```python
from build123d import *

# Parameters (mm, degrees)
SKETCH10_W          = 150
SKETCH10_H          = 150
BOSS_EXTRUDE3_DEPTH = 10
SKETCH12_W          = 100
SKETCH12_H          = 37.5
CUT_EXTRUDE2_DEPTH  = 10
FILLET7_R           = 10


with BuildPart() as part:
    # Sketch10 → Boss-Extrude3 (new body)
    with BuildSketch(Plane(origin=(0, 0, 0), x_dir=(0, 0, -1), z_dir=(1, 0, 0))):
        with Locations((75, 112.5)):
            Rectangle(SKETCH10_W, SKETCH10_H)
    extrude(amount=BOSS_EXTRUDE3_DEPTH)

    # Sketch12 → Cut-Extrude2 (cut)
    with BuildSketch(Plane.ZY):
        with Locations((-75, 56.25)):
            Rectangle(SKETCH12_W, SKETCH12_H)
    extrude(amount=-CUT_EXTRUDE2_DEPTH, mode=Mode.SUBTRACT)

    # Fillet7
    fillet7_edges = [part.edges().sort_by_distance(p)[0] for p in [
        (5, 37.5, -125),
        (5, 37.5, -25),
        (5, 187.5, 0),
        (5, 187.5, -150),
        (5, 37.5, -150),
        (5, 37.5, 0),
    ]]
    fillet(fillet7_edges, radius=FILLET7_R)


solid = part.part
```
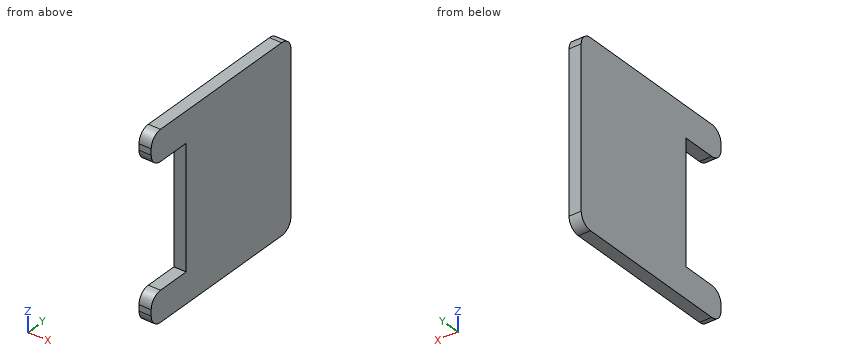
Build history of the part. All positions in model axes, mm. Give positions to 0.01 mm unless a question says otherwise; leave off trailing zeros. Loops run counter-clockwise (first coordinate to the right, second up) from the corner with the lowest first, then second, coordinate; pieces in that order, holes last.
Item 1: Drill centre lines: line 1 (Y direction, x = 4.25, z = -31); line 2 (Z direction, x = 2.25, y = 70.5); line 3 (Y direction, x = 5, z = -16.5). Where is each one in solid material? Low to high.
Answers follow:
line 1: y = 75 to 187.5
line 2: z = -150 to -125, -25 to 0
line 3: y = 37.61 to 187.5
Item 2: Flat gauge pin, fed straight in: pin 1 (3 mm diameter, centred on x = 2, z = -17, fed in from -Y). Where does the tip first touch, or does it go through?
Answers follow:
pin 1: stops at y = 37.51
Item 3: Slice it at B-B, the plane z = -74. List the corners of the cut face in (x, y), and give its area (4 significant figures).
Answers follow:
outline: (0, 75) - (10, 75) - (10, 187.5) - (0, 187.5) - close
area: 1,125 mm2
Item 4: Slice it at A-A, the plane x = 2.5. List the corners of the cut face in (y, z), and give its area (3 significant figures).
Answers follow:
outline: (37.5, -140) arc R10 ccw to (47.5, -150) - (177.5, -150) arc R10 ccw to (187.5, -140) - (187.5, -10) arc R10 ccw to (177.5, 0) - (47.5, 0) arc R10 ccw to (37.5, -10) - (37.5, -15) arc R10 ccw to (47.5, -25) - (75, -25) - (75, -125) - (47.5, -125) arc R10 ccw to (37.5, -135) - close
area: 18,600 mm2
